from build123d import *

# Parameters (mm, degrees)
SKETCH_1_W          = 20
SKETCH_1_H          = 20
SKETCH_1_W_2        = 18
SKETCH_1_H_2        = 18
EXTRUDE_1_DEPTH     = 297.5
SKETCH_2_R          = 3
CUT_EXTRUDE_1_DEPTH = 10
SKETCH_4_R          = 2
CUT_EXTRUDE_3_DEPTH = 10
CUT_EXTRUDE_4_DEPTH = 10


with BuildPart() as part:
    # 草图1 → 凸台-拉伸1 (new, symmetric)
    with BuildSketch(Plane.XY):
        Rectangle(SKETCH_1_W, SKETCH_1_H)
        Rectangle(SKETCH_1_W_2, SKETCH_1_H_2, mode=Mode.SUBTRACT)
    extrude(amount=EXTRUDE_1_DEPTH, both=True)

    # 草图2 → 切除-拉伸1 (cut)
    with BuildSketch(Plane(origin=(0, 10, 0), x_dir=(1, 0, 0), z_dir=(0, 1, 0))):
        with Locations(Location((0, -287.5, 0), (0, 0, 270))):
            Circle(SKETCH_2_R)
    cut_extrude_1 = extrude(amount=-CUT_EXTRUDE_1_DEPTH, mode=Mode.SUBTRACT)

    # 镜向1: 切除-拉伸1 across plane
    add(cut_extrude_1.mirror(Plane.XY), mode=Mode.SUBTRACT)

    # 草图4 → 切除-拉伸3 (cut)
    with BuildSketch(Plane(origin=(0, -9, 0), x_dir=(1, 0, 0), z_dir=(0, 1, 0))):
        with Locations(Location((0, -79, 0), (0, 0, 270))):
            Circle(SKETCH_4_R)
        with Locations(Location((0, -61, 0), (0, 0, 270))):
            Circle(SKETCH_4_R)
    cut_extrude_3 = extrude(amount=-CUT_EXTRUDE_3_DEPTH, mode=Mode.SUBTRACT)

    # 草图5 → 切除-拉伸4 (cut)
    with BuildSketch(Plane.XZ.offset(-9)):
        with BuildLine():
            Line((4.2, 79), (4.2, 61))
            ThreePointArc((4.2, 61), (0, 56.8), (-4.2, 61))
            Line((-4.2, 61), (-4.2, 79))
            ThreePointArc((-4.2, 79), (0, 83.2), (4.2, 79))
        make_face()
    cut_extrude_4 = extrude(amount=-CUT_EXTRUDE_4_DEPTH, mode=Mode.SUBTRACT)

    # 镜向2: 切除-拉伸3, 切除-拉伸4 across plane
    add(cut_extrude_3.mirror(Plane.XY), mode=Mode.SUBTRACT)
    add(cut_extrude_4.mirror(Plane.XY), mode=Mode.SUBTRACT)


solid = part.part
Could you check a few things on this model? Use its own coordinates, in mm. A direction names the side the tool comes from. Coordinates: 2 decimals unless noted, no trailing zeros. Loops run counter-clockwise (first coordinate to the right, second up) from the corner with the lowest first, then second, coordinate; pieces in that order, holes last.
1. I need wall thicknesses on L1, parallel to Y at x = -4.25, z = 23; L2, parallel to X at y = -9.5, z = -61. Which ranges of each line are inside material? Lowest first, please.
2. We'd pull the mould along X, two halves only. Please class faces 1 (the face through (-10, 0, 4)), 2 (the face through (-0.8, -9.6, 297.5)), 3 (the face through (0, 9, 4)): released by +X, released by -X, zero draft, split by the parting line, or undercut.
3. Imagine slicing it at A-A (y = -1.5). Please give me the cut outline in (x, z), and give its area (3 significant figures).
4. For P1, Ø3.5, axis at x = 0, z = -61, coming from the +Y side; P2, Ø6.5, axis at x = 0, z = -79, coming from the +Y side, each with a flat end and sliding along its axis, tell me the tip position at first contact or that it passes through.
5. For faces 4 (the face through (-0.8, -9.6, -297.5)), 5 (the face through (9, 0, 4)), which set-ups out of +Z, -Z, +X, -X, +Y, -Y let a thin tool reach every point of the face, with its end or its side?
6. Imagine slicing it at B-B (z = 90.5). Please give me the cut outline in (x, y).
Computed values:
1. L1: y = -10 to -9, 9 to 10
1. L2: x = -10 to -2, 2 to 10
2. face 1: released by -X
2. face 2: zero draft
2. face 3: undercut
3. outline: (-10, -297.5) - (-9, -297.5) - (-9, 297.5) - (-10, 297.5) - close; (9, -297.5) - (10, -297.5) - (10, 297.5) - (9, 297.5) - close
3. area: 1,190 mm2
4. P1: passes through
4. P2: stops at y = -9
5. face 4: -Z, +X, -X, +Y, -Y
5. face 5: +Z, -Z
6. outline: (-10, -10) - (10, -10) - (10, 10) - (-10, 10) - close; hole (-9, -9) - (9, -9) - (9, 9) - (-9, 9) - close
